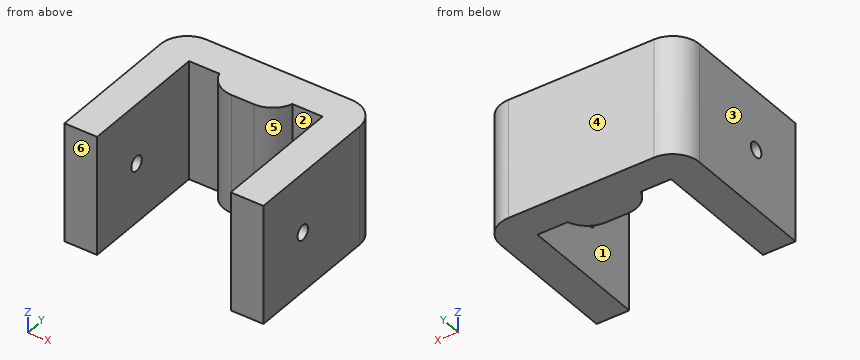
from build123d import *

# Parameters (mm, degrees)
BOSS_EXTRUDE1_DEPTH = 20
FILLET1_R           = 4.5
FILLET2_R           = 4.5
SKETCH2_R           = 1.25
CUT_EXTRUDE1_DEPTH  = 48.618693808


with BuildPart() as part:
    # Sketch1 → Boss-Extrude1 (new body)
    with BuildSketch(Plane.XY):
        Polygon((-16.75, 0), (-16.75, 27.3), (16.75, 27.3), (16.75, 0), (11.25, 0), (11.25, 21.8), (6.15, 21.8), (6.15, 18.7), (-6.15, 18.7), (-6.15, 21.8), (-11.25, 21.8), (-11.25, 0), align=None)
    extrude(amount=BOSS_EXTRUDE1_DEPTH)

    # Fillet1
    fillet1_edges = [part.edges().sort_by_distance(p)[0] for p in [
        (16.75, 27.3, 10),
        (-16.75, 27.3, 10),
    ]]
    fillet(fillet1_edges, radius=FILLET1_R)

    # Fillet2
    # the kernel refuses this fillet: 4.5 mm, written as the material it takes off along each edge
    with BuildSketch(Plane(origin=(-6.15, 18.7, -10.69170239), x_dir=(0, 1, 0), z_dir=(0, 0, 1))) as fillet2_piece_1:
        with BuildLine():
            CenterArc((4.5, -4.276680956), FILLET2_R, 108.126203961, 71.873796039)
            Line((0, -4.276680956), (-0.09, -4.276680956))
            Line((-0.09, -4.276680956), (-0.09, 0))
            Line((-0.09, 0), (0, 0.09))
            ThreePointArc((0, 0.09), (1.55, 0.09), (3.072, 0.085533619))
            Line((3.072, 0.085533619), (3.1, 0))
        make_face()
    extrude(amount=41.38340478, mode=Mode.SUBTRACT)
    with BuildSketch(Plane(origin=(6.15, 18.7, -10.69170239), x_dir=(-1, 0, 0), z_dir=(0, 0, 1))) as fillet2_piece_2:
        with BuildLine():
            CenterArc((4.276680956, -4.5), FILLET2_R, 90, 71.873796039)
            Line((0, -3.1), (-0.085533619, -3.072))
            ThreePointArc((-0.085533619, -3.072), (-0.09, -1.55), (-0.09, 0))
            Line((-0.09, 0), (0, 0.09))
            Line((0, 0.09), (4.276680956, 0.09))
            Line((4.276680956, 0.09), (4.276680956, 0))
        make_face()
    extrude(amount=41.38340478, mode=Mode.SUBTRACT)

    # Sketch2 → Cut-Extrude1 (cut, through all)
    with BuildSketch(Plane(origin=(16.75, 0, 0), x_dir=(0, 0, -1), z_dir=(1, 0, 0))):
        with Locations(Location((-10, 9.35, 0), (0, 0, 90))):
            Circle(SKETCH2_R)
    extrude(amount=-CUT_EXTRUDE1_DEPTH, mode=Mode.SUBTRACT)


solid = part.part
Design review of the part built by this model. Coordinates are the model's own, in mm. Face numbers are marked on the shaded views. A direction names the side the tool comes from. Give positions to 0.01 mm unless a question says otherwise; leave off trailing zeros. Write each loop counter-clockwise with the first axis right and the second up, starting at its lowest first coordinate (ties: lowest second). Pieces come first, ordered by that corner, then holes. Notation, with made-up numbers: M -35,55 L 7,55 A25 cw 7,93 Z; hole C -33.75,28.5 d1. An arc over 180 degrees is marked long. Return JSON: item names as keys, results as strings. Group by question number.
Item 1: Take a section at A-A (z = 10). Give the boundary of the cut face in (x, y).
Item 2: Take a section at B-B (y = 5.5). Give the boundary of the cut face in (x, z).
Item 3: Take a section at C-C (y = 9.35). Give the boundary of the cut face in (x, z).
Item 4: The part is to be moulded in two halves that separate along X. For the marked faces 1, 2, 3 and 4, say which applies: pulls with the +X half, pulls with the -X half, needs draft (parallel to the pull), parting line crosses it, or undercut.
Item 5: Tool access review of the marked faces 5 and 6: name each direction out of +Z, -Z, +X, -X, +Y, -Y from which nothing blocks a thin tool from reaching the whole face with its end or side.
Item 6: Wall thickness on line 1 along X through (y, z) = (8, 18.75); line 2 along Z through (x, y) = (14.65, 9.35); line 3 along X through (y, z) = (20, 12.25): over which ranges is each line inside the solid? List them lowest first.
Item 7: Clearance check with flat-ended pins moving along their axes: pin 1 Ø1.1 at (x, z) = (-0.5, 9) entering from -Y; pin 2 Ø2.5 at (x, z) = (7.5, 9.5) entering from -Y. State where each tip first meets the part, or that it passes through.
Item 8: Take a section at D-D (z = 6.75). Give the boundary of the cut face in (x, y), plus the area to 3 significant figures.
Return value:
{
 "1": {"outline": "M -16.75,0 L -11.25,0 L -11.25,8.1 L -16.75,8.1 Z; M -16.75,10.6 L -11.25,10.6 L -11.25,21.8 L -6.15,21.8 A4.5 ccw -1.87,18.7 L 1.87,18.7 A4.5 ccw 6.15,21.8 L 11.25,21.8 L 11.25,10.6 L 16.75,10.6 L 16.75,22.8 A4.5 ccw 12.25,27.3 L -12.25,27.3 A4.5 ccw -16.75,22.8 Z; M 11.25,0 L 16.75,0 L 16.75,8.1 L 11.25,8.1 Z"},
 "2": {"outline": "M -16.75,0 L -11.25,0 L -11.25,20 L -16.75,20 Z; M 11.25,0 L 16.75,0 L 16.75,20 L 11.25,20 Z"},
 "3": {"outline": "M -16.75,0 L -11.25,0 L -11.25,8.75 L -16.75,8.75 Z; M -16.75,11.25 L -11.25,11.25 L -11.25,20 L -16.75,20 Z; M 11.25,0 L 16.75,0 L 16.75,8.75 L 11.25,8.75 Z; M 11.25,11.25 L 16.75,11.25 L 16.75,20 L 11.25,20 Z"},
 "4": {"face 1": "undercut", "face 2": "undercut", "face 3": "pulls with the -X half", "face 4": "needs draft"},
 "5": {"face 5": "+Z, -Z, -Y", "face 6": "+Z, -Z, +X, -X, -Y"},
 "6": {"line 1": "x = -16.75 to -11.25, 11.25 to 16.75", "line 2": "z = 0 to 8.75, 11.25 to 20", "line 3": "x = -16.75 to -11.25, -5.04 to 5.04, 11.25 to 16.75"},
 "7": {"pin 1": "stops at y = 18.7", "pin 2": "stops at y = 21.8"},
 "8": {"outline": "M -16.75,0 L -11.25,0 L -11.25,21.8 L -6.15,21.8 A4.5 ccw -1.87,18.7 L 1.87,18.7 A4.5 ccw 6.15,21.8 L 11.25,21.8 L 11.25,0 L 16.75,0 L 16.75,22.8 A4.5 ccw 12.25,27.3 L -12.25,27.3 A4.5 ccw -16.75,22.8 Z", "area": "446 mm2"}
}
